from build123d import *

# Parameters (mm, degrees)
BOSS_EXTRUDE1_DEPTH = 5.5626
SKETCH2_R           = 3.175
CUT_EXTRUDE1_DEPTH  = 34.158539907


with BuildPart() as part:
    # Sketch1 → Boss-Extrude1 (new, symmetric)
    with BuildSketch(Plane(origin=(0, 0, 0), x_dir=(1, 0, 0), z_dir=(0, 1, 0))):
        with BuildLine():
            Line((-12.7, 0), (-28.575, 0))
            Line((-28.575, 0), (-28.575, 15.875))
            Line((-28.575, 15.875), (28.575, 15.875))
            Line((28.575, 15.875), (28.575, 0))
            Line((28.575, 0), (12.7, 0))
            ThreePointArc((12.7, 0), (0, 12.7), (-12.7, 0))
        make_face()
        with BuildLine():
            Line((16.1925, 14.605), (7.540207225, 14.605))
            ThreePointArc((7.540207225, 14.605), (6.924551883, 14.125542599), (7.238598936, 13.4112))
            ThreePointArc((7.238598936, 13.4112), (12.258915713, 9.054092199), (14.946923077, 2.974405913))
            ThreePointArc((14.946923077, 2.974405913), (16.317033746, 1.958393589), (17.4625, 3.222273072))
            Line((17.4625, 3.222273072), (17.4625, 13.335))
            ThreePointArc((17.4625, 13.335), (17.090525612, 14.233025612), (16.1925, 14.605))
        make_face(mode=Mode.SUBTRACT)
        with BuildLine():
            Line((-17.4625, 3.222273072), (-17.4625, 13.335))
            ThreePointArc((-17.4625, 13.335), (-17.090525612, 14.233025612), (-16.1925, 14.605))
            Line((-16.1925, 14.605), (-7.540207225, 14.605))
            ThreePointArc((-7.540207225, 14.605), (-6.924551883, 14.125542599), (-7.238598936, 13.4112))
            ThreePointArc((-7.238598936, 13.4112), (-12.258915713, 9.054092199), (-14.946923077, 2.974405913))
            ThreePointArc((-14.946923077, 2.974405913), (-16.317033746, 1.958393589), (-17.4625, 3.222273072))
        make_face(mode=Mode.SUBTRACT)
    extrude(amount=BOSS_EXTRUDE1_DEPTH, both=True)

    # Sketch2 → Cut-Extrude1 (cut, through all)
    with BuildSketch(Plane.XY):
        with Locations((-22.225, 0)):
            Circle(SKETCH2_R)
        with Locations((22.225, 0)):
            Circle(SKETCH2_R)
    extrude(amount=-CUT_EXTRUDE1_DEPTH, mode=Mode.SUBTRACT)


solid = part.part
Build history of the part. All positions in model axes, mm. A direction names the side the tool comes from. Coordinates: 2 decimals unless noted, no trailing zeros. Order: outer loops, then holes, each group sorted by start corner. A loop starts at its lowest first (then second) coordinate and runs counter-clockwise, first axis right, second up. Notation, with made-up numbers: M -26.75,48.25 L 27.25,48.25 A31 ccw 27.25,87.25 Z; hole C -1,7 d3. An arc over 180 degrees is marked long. One line per question, with ' | ' between items. Start each with the question number.
Q1. Saw through at B-B (z = -14). List the corners of the cut face in (x, y) (3 decimals), then the cut area to 3 significant figures.
Q2. Two-plate mould, pull along X, no slides. Class faces 3 (the face through (0, 0, -15.875)), 4 (the face through (28.575, 0, -8)), 5 (the face through (-17.1, 0.078, -14.223)): +X half, -X half, draft (parallel to the pull), parting line (faces both ways), or undercut.
Q3. Saw through at A-A (y = 0). Count the separate pieces of the cut face and the enclosed holes in it, then the cut area to 3 significant figures.
Q4. Probe L1, parallel to X at y = 1.25, z = -11.25 (1 decimal); L2, parallel to X at y = 0.75, z = -6.5 (1 decimal); L3, parallel to X at y = -0.25, z = -13.5 (3 decimals). List the from-to ranges inside material, lowest first. Write a range as from..to.
Q5. Saw through at D-D (x = 23). List the corners of the cut face in (y, z) (3 decimals).
Q6. Saw through at C-C (y = -3.75). List the corners of the cut face in (x, z) (1 decimal).
Q7. 3-axis set-ups, long thin cutter, end or side, ignore diameter. For faces 1 (the face through (0.279, 0.078, -12.697)), 2 (the face through (17.462, 0, -8)): which of +Z, -Z, +X, -X, +Y, -Y reach the whole face in a straight line?
Q8. Flat gauge pins, fed straight in: pin 1 Ø1 at (x, y) = (-22.5, -2) entering from +Z; pin 2 Ø4.5 at (x, y) = (-10.5, 0) entering from +Z. Where does each tip first touch, or does it go through?
Check values:
1) outline: M -28.575,-5.563 L -17.274,-5.563 L -17.274,5.563 L -28.575,5.563 Z; M -6.906,-5.563 L 6.906,-5.563 L 6.906,5.563 L -6.906,5.563 Z; M 17.274,-5.563 L 28.575,-5.563 L 28.575,5.563 L 17.274,5.563 Z; hole C -22.225,0 d6.35; hole C 22.225,0 d6.35 | area: 342 mm2
2) face 3: draft | face 4: +X half | face 5: undercut
3) separate pieces: 3 | enclosed holes: 2 | area: 317 mm2
4) L1: x = -28.6..-25.1, -19.3..-17.5, -10.3..-5.9, 5.9..10.3, 17.5..19.3, 25.1..28.6 | L2: x = -28.6..-25.3, -19.1..-17.5, -13.8..-10.9, 10.9..13.8, 17.5..19.1, 25.3..28.6 | L3: x = -28.575..-25.39, -19.06..-17.452, -7.113..7.113, 17.452..19.06, 25.39..28.575
5) outline: M -5.563,-15.875 L -3.079,-15.875 L -3.079,0 L -5.563,0 Z; M 3.079,-15.875 L 5.563,-15.875 L 5.563,0 L 3.079,0 Z
6) outline: M -28.6,-15.9 L 28.6,-15.9 L 28.6,0 L 12.7,0 A12.7 cw -12.7,0 L -28.6,0 Z; hole M -17.5,-13.3 A1.3 ccw -16.2,-14.6 L -7.5,-14.6 A0.6 ccw -7.2,-13.4 A15.2 cw -14.9,-3 A1.3 ccw -17.5,-3.2 Z; hole M 7.2,-13.4 A0.6 ccw 7.5,-14.6 L 16.2,-14.6 A1.3 ccw 17.5,-13.3 L 17.5,-3.2 A1.3 ccw 14.9,-3 A15.2 cw Z
7) face 1: +Z, +Y, -Y | face 2: +Y, -Y
8) pin 1: passes through | pin 2: stops at z = 0
